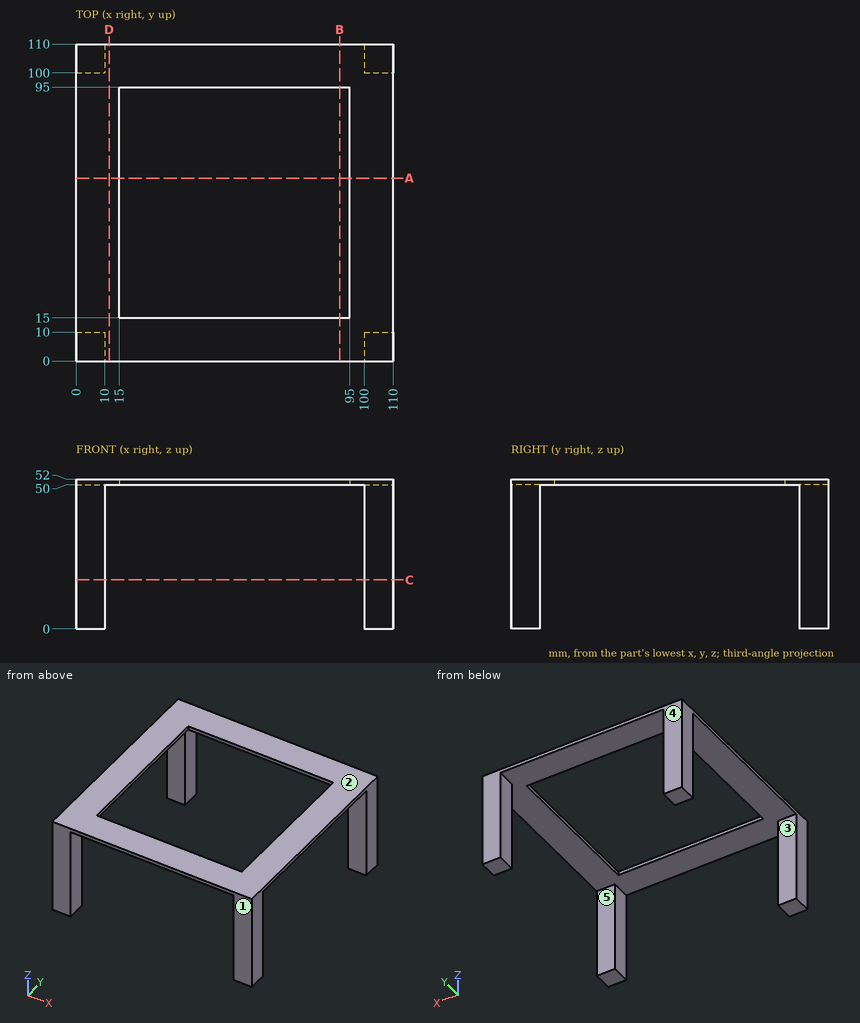
Here's the drawing with two shaded views (mm, measured from the low corner). I have some questions. A direction names the side the tool comes from. Give positions to 0.01 mm unless a question says otherwise; leave off trailing zeros. Loops run counter-clockwise (first coordinate to the right, second up) from the corner with the lowest first, then second, coordinate; pieces in that order, holes last. Notation, with made-up numbers: M 49,84.5 L 84,84.5 A7 cw 84,92.5 Z; hole C -24,43.5 d11. An arc over 180 degrees is marked long. Use one line per item in the form item = value. Start each with the question number.
(1) I want a section at C-C, the plane z = 17. Write out the boundary of the cut face in (x, y).
(2) I want a section at D-D, the plane x = 11.5. Write out the boundary of the cut face in (y, z).
(3) I'm going to push a flat-ended pin straight in: P1, Ø11, axis at y = 104, z = 20, coming from the -X side. Where does the tip first touch, or does it pass through?
(4) On a 3-axis mill with a long thin cutter (end or side, diameter ignored), from which of +Z, -Z, +X, -X, +Y, -Y can I reach the whole of each face in a straight line? I mean the marked faces 4 and 5. Say none if no direction works.
(5) I want a section at A-A, the plane y = 63.5. Write out the boundary of the cut face in (x, z).
(6) Thinking about a two-plate mould opening in Y: for the marked faces 1, 2 and 3, which applies, released by +Y, released by -Y, zero draft, split by the parting line, or undercut?
(7) Please list where these lines run through material, in increasing order: line 1 (X direction, y = 8, z = 37); line 2 (Z direction, x = 100, y = 21).
Worked out:
q1.outline = M 0,0 L 10,0 L 10,10 L 0,10 Z; M 0,100 L 10,100 L 10,110 L 0,110 Z; M 100,0 L 110,0 L 110,10 L 100,10 Z; M 100,100 L 110,100 L 110,110 L 100,110 Z
q2.outline = M 0,50 L 110,50 L 110,52 L 0,52 Z
q3.P1 = 0
q4.face_4 = +Z, -Z, +X, -X, +Y
q4.face_5 = -Z, +X, -X
q5.outline = M 0,50 L 15,50 L 15,52 L 0,52 Z; M 95,50 L 110,50 L 110,52 L 95,52 Z
q6.face_1 = released by -Y
q6.face_2 = zero draft
q6.face_3 = undercut
q7.line_1 = 0 to 10, 100 to 110
q7.line_2 = 50 to 52
